Check sheet for the modelled part. Datum: model origin and axes. Units: mm. A direction names the side the tool comes from. Give positions to 0.01 mm unless a question says otherwise; leave off trailing zeros. Write each loop counter-clockwise with the first axis right and the second up, starting at its lowest first coordinate (ties: lowest second). Pieces come first, ordered by that corner, then holes. Notation, with made-up numbers: (8, 20.25) -> (26, 20.25) arc R13 ccw to (26, 41.25) -> close; hole circle Ø10 at (6, 2.25). An arc over 180 degrees is marked (long way). Return JSON: item names as keys, results as strings.
Autodesk Inventor part; units mm, degrees
ref_plane "YZ Plane" through (0, 0, 0) normal (1, 0, 0) x (0, 1, 0)
ref_plane "XZ Plane" through (0, 0, 0) normal (0, 1, 0) x (-1, 0, 0)
ref_plane "XY Plane" through (0, 0, 0) normal (0, 0, 1) x (1, 0, 0)
sketch "Boceto1" plane through (0, 0, 0) normal (0, 1, 0) x (-1, 0, 0)
  circle A0 centre (0, 0) radius 51
  circle A1 centre (0, 0) radius 30
  circle A2 centre (0, 0) radius 52
  point P0 (41.233, 0)
  point P1 (29.1561, 29.1561)
  point P2 (0, 41.233)
  point P3 (-29.1561, 29.1561)
  point P4 (-41.233, 0)
  point P5 (-29.1561, -29.1561)
  point P6 (0, -41.233)
  point P7 (29.1561, -29.1561)
  dimension "d0" = 102
  dimension "d1" = 60
  dimension "d2" = 41.233
  dimension "d3" = 1
  dimension "d8" = 360
extrude "Extrusión1" add sketch "Boceto1" along normal blind 1 contours A0
extrude "Extrusión2" add sketch "Boceto1" along normal blind 152 contours A0 | A2
sketch "Boceto3" plane through (0, 152, 0) normal (0, 1, 0) x (1, 0, 0)
  circle A0 centre (0, 0) radius 30
extrude "Extrusión4" add sketch "Boceto3" against normal blind 151
shell "Vaciado1" thickness 1 removed faces 1 at (-8.8546, 1, 4.6472)
fillet "Empalme1" radius 8 2 edges at (51, 151, 0) (52, 152, 0)
hole "Hole1" at (-41.233, 0, 0) at (-29.1561, 0, 29.1561) at (0, 0, 41.233) at (29.1561, 0, 29.1561) at (41.233, 0, 0) at (29.1561, 0, -29.1561) at (0, 0, -41.233) at (-29.1561, 0, -29.1561) direction (0, 1, 0) diameter 3 depth 8 tip angle 118
properties part number "Capa" material "Caucho, Silicona"
(1) Cross-section at A-A on y = 15.5. Enter the section's corners in (x, z).
Reply:
{"outline": "circle Ø104 at (0, 0); hole circle Ø102 at (0, 0)"}
(2) Thickness scan on L1, parallel to Z at x = 0, y = 0.3; L2, parallel to Z at x = 1, y = 125; L3, parallel to Y at x = -35, z = 16. Record the ranges inside material, lowest first.
Reply:
{"L1": "-52 to -42.73, -39.73 to -30, 30 to 39.73, 42.73 to 52", "L2": "-51.99 to -50.99, 50.99 to 51.99", "L3": "0 to 1, 151 to 152"}
(3) Depth check by flat-ended pin: pin 1 Ø1 at (y, z) = (128, -4.5) entering from +X; pin 2 Ø8 at (y, z) = (29.5, -13.5) entering from +X; pin 3 Ø1.5 at (y, z) = (115, 4) entering from -X. Enter the tip coordinate at first touch or a pass-through.
Reply:
{"pin 1": "x = 51.85", "pin 2": "x = 51.12", "pin 3": "x = -51.9"}
(4) Release check for a two-part mould opening along Z. For faces 1 (the flat face through (-1, 152, -1)), 2 (the cylindrical face through (11.056, 71.006, 49.787)), 3 (the cylindrical face through (41.265, 70.992, 31.641)) record: pulls with the +Z half, pulls with the -Z half, needs draft (parallel to the pull), parting line crosses it, or undercut.
Reply:
{"face 1": "needs draft", "face 2": "undercut", "face 3": "parting line crosses it"}
(5) Set-up check for faces 4 (the flat face through (-22, 0, -22)), 5 (the cylindrical face through (29.97, 0.49, -1.32)), 6 (the flat face through (-1, 151, -1)): record each of +Z, -Z, +X, -X, +Y, -Y from which the full face is reachable in a straight line by a thin tool's end or side.
Reply:
{"face 4": "+Z, -Z, +X, -X, -Y", "face 5": "-Y", "face 6": "none"}
